Geometry check sheet. Reference: the model listing, model coordinates, mm. Coordinates: 2 decimals unless noted, no trailing zeros. Order: outer loops, then holes, each group sorted by start corner. A loop starts at its lowest first (then second) coordinate and runs counter-clockwise, first axis right, second up. Notation, with made-up numbers: (22, 24) - (29, 24) arc R16 ccw to (29, 33) - close; hole circle Ø1 at (8.25, 89). An arc over 180 degrees is marked (long way). Return JSON: item names as keys, results as strings. Group by question number.
Item 1: Gauge pin test, flat ends, axial feed: pin 1 (6 mm diameter, centred on x = -4, y = -5, fed in from +Z); pin 2 (3 mm diameter, centred on y = 3.5, z = -14.5, fed in from -X); pin 3 (6 mm diameter, centred on x = 1.5, z = 1, fed in from +Y); pin 4 (5 mm diameter, centred on x = -3, y = 3, fed in from -Z). Record the tip position at first contact, or that the pin passes through.
Item 2: Section check C-C on z = 3.5. Enter the section's corners in (x, y), then the cut area to 3 significant figures.
Item 3: Scan lines: probe 1 along X at (y, z) = (-0.25, -4.5); probe 2 along Z at (x, y) = (1.5, -2.5); probe 3 along X at (y, z) = (-4.5, 19). Record each from-to range of solid material in increasing order.
Item 4: Section check A-A on x = 0. Enter the section's corners in (y, z), then the cut area to 3 significant figures.
Item 5: Section check D-D on z = 22.5. Enter the section's corners in (x, y), then the cut area to 3 significant figures.
from build123d import *

# Parameters (mm, degrees)
F0_R     = 6.35
F1_DEPTH = 25.4
F2_R     = 6.35


with BuildPart() as f1:
    # F0 (on Top) → F1 (new body)
    with BuildSketch(Plane.XY):
        Circle(F0_R)
    extrude(amount=F1_DEPTH)

    # F2
    f2_edges = [f1.edges().sort_by_distance(p)[0] for p in [
        (-6.35, 0, 25.4),
    ]]
    fillet(f2_edges, radius=F2_R)

    # F3: F1 across face


with BuildPart() as f1_1:
    add(f1.part)
    add(f1.part.mirror(Plane(origin=(0, 0, 0), x_dir=(1, 0, 0), z_dir=(0, 0, -1))))


solid = f1_1.part
Computed:
{
 "1": {"pin 1": "stops at z = 24.41", "pin 2": "stops at x = -6.03", "pin 3": "stops at y = 6.35", "pin 4": "stops at z = -25.16"},
 "2": {"outline": "circle Ø12.7 at (0, 0)", "area": "127 mm²"},
 "3": {"probe 1": "x = -6.35 to 6.35", "probe 2": "z = -24.69 to 24.69", "probe 3": "x = -4.48 to 4.48"},
 "4": {"outline": "(-6.35, -19.05) arc R6.35 ccw to (6.35, -19.05) - (6.35, 19.05) arc R6.35 ccw to (-6.35, 19.05) - close", "area": "611 mm²"},
 "5": {"outline": "circle Ø10.66 at (0, 0)", "area": "89.3 mm²"}
}
